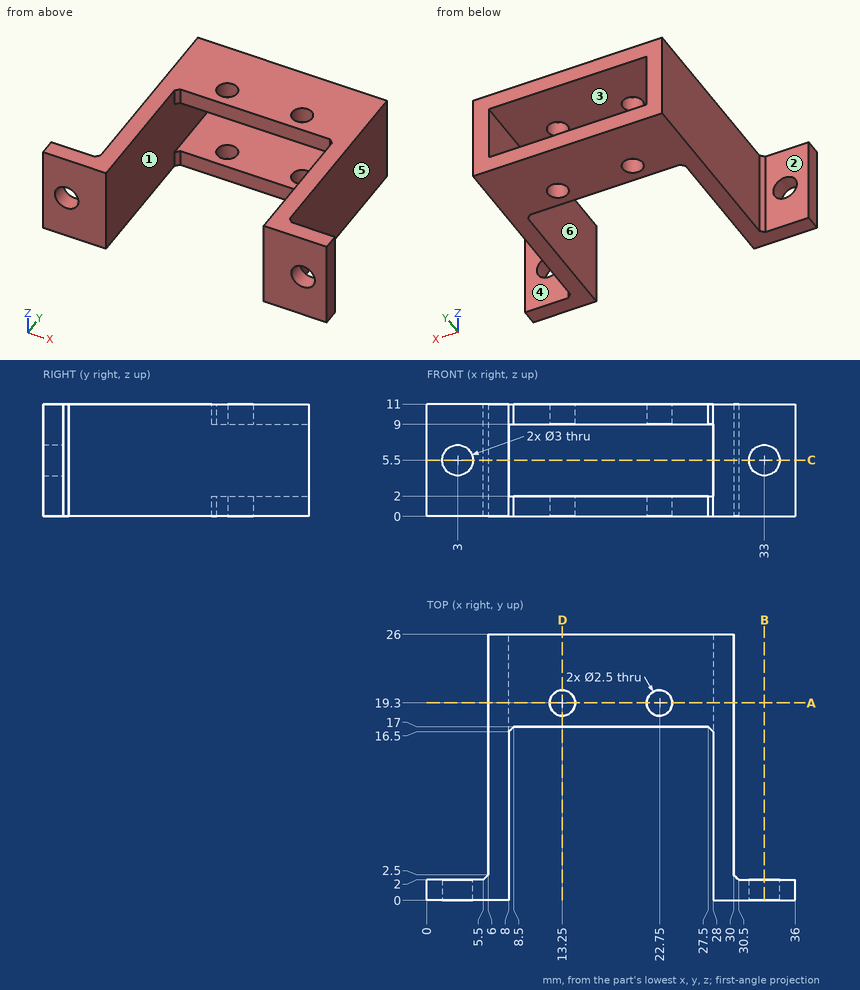
Geometry: see drawing. Coordinates: mm, zero at the bounding-box minimum. A direction names the side the tool comes from. Round coordinates to 2 decimals unless told otherwise and drop trailing zeros. Write each loop counter-clockwise with the first axis right and the second up, starting at its lowest first coordinate (ties: lowest second). Pieces come first, ordered by that corner, then holes.
Item 1: Pin query (flat end, axial travel): P1, Ø3.5, axis at x = 3, z = 5.5, coming from the +Y side; P2, Ø2, axis at x = 15.5, z = 0.5, coming from the -Y side; P3, Ø5, axis at y = 12, z = 3.5, coming from the -X side. Return the tip coordinate at first contact, or that it passes through.
Item 2: Section query D-D (x = 13.25). Return loops of the section in (y, z).
Item 3: Section query A-A (y = 19.3). Return loops of the section in (x, z).
Item 4: Section query C-C (z = 5.5). Return loops of the section in (x, y), plus the area to 3 significant figures.
Item 5: Section query B-B (x = 33). Return loops of the section in (y, z).
Item 6: Mould query, pull axis X, two halves, no side actions, for the marked faces 4, 5 and 6. Classes: +X half, -X half, draft (parallel to the pull), parting line (faces both ways), or undercut.
Item 7: Set-up query: the marked faces 1, 2 and 3. Return all of +Z, -Z, +X, -X, +Y, -Y with unobstructed straight access to the full face (end or side cutting, diameter ignored); none if empty.
Item 8: Material intervals for L1, parallel to X at y = 12.75, z = 1; L2, parallel to Y at x = 13.25, z = 0.75; L3, parallel to Z at x = 24, y = 18.5, sorted ascending.
Completed:
1. P1: stops at y = 2
1. P2: stops at y = 17
1. P3: stops at x = 6
2. outline: (17, 0) - (18.05, 0) - (18.05, 2) - (17, 2) - close; (17, 9) - (18.05, 9) - (18.05, 11) - (17, 11) - close; (20.55, 0) - (26, 0) - (26, 2) - (20.55, 2) - close; (20.55, 9) - (26, 9) - (26, 11) - (20.55, 11) - close
3. outline: (6, 0) - (12, 0) - (12, 2) - (8, 2) - (8, 9) - (12, 9) - (12, 11) - (6, 11) - close; (14.5, 0) - (21.5, 0) - (21.5, 2) - (14.5, 2) - close; (14.5, 9) - (21.5, 9) - (21.5, 11) - (14.5, 11) - close; (24, 0) - (30, 0) - (30, 11) - (24, 11) - (24, 9) - (28, 9) - (28, 2) - (24, 2) - close
4. outline: (0, 0) - (1.5, 0) - (1.5, 2) - (0, 2) - close; (4.5, 0) - (8, 0) - (8, 26) - (6, 26) - (6, 2.5) - (5.5, 2) - (4.5, 2) - close; (28, 0) - (31.5, 0) - (31.5, 2) - (30.5, 2) - (30, 2.5) - (30, 26) - (28, 26) - close; (34.5, 0) - (36, 0) - (36, 2) - (34.5, 2) - close
4. area: 116 mm2
5. outline: (0, 0) - (2, 0) - (2, 4) - (0, 4) - close; (0, 7) - (2, 7) - (2, 11) - (0, 11) - close
6. face 4: draft
6. face 5: +X half
6. face 6: undercut
7. face 1: -Y
7. face 2: +Z, -Z, -X, +Y
7. face 3: +Y, -Y
8. L1: x = 6 to 8, 28 to 30
8. L2: y = 17 to 18.05, 20.55 to 26
8. L3: z = 0 to 2, 9 to 11
